Work out the finished part from the listing and answer in its coordinate system (mm). A direction names the side the tool comes from. Round coordinates to 2 decimals unless told otherwise and drop trailing zeros. Loops run counter-clockwise (first coordinate to the right, second up) from the corner with the lowest first, then second, coordinate; pieces in that order, holes last. Notation, with made-up numbers: (6.25, -30.5) - (53.25, -30.5) arc R20 cw to (53.25, -22.5) - close; hole circle Ø3 at (-35.5, 17). An arc over 180 degrees is marked (long way). Answer as CSV lines item,"result". Start each with the question number.
Q1. Straight lines are drawn through the part: L1, parallel to Y at x = 5, z = -14.05; L2, parallel to X at y = 10.5, z = -11; L3, parallel to Z at x = 2.75, y = 6.75. For each, find the intervals that lie inside material, in ascending order. Write a range as [from, to].
Q2. Section A-A on x = 5 is taken. Write down the section's boundary in (y, z).
Q3. Each of these flat-tipped pins is pushed along its axis until it touches: pin 1 Ø4.5 at (x, z) = (5.5, -9) entering from -Y; pin 2 Ø2.5 at (x, z) = (5, -11) entering from +Y; pin 3 Ø2 at (y, z) = (12, -6) entering from -X; pin 4 Ø1.2 at (x, y) = (5, 12) entering from -Z. Where does it stop, or does it pass through?
Q4. Section B-B on z = -11 is taken. Write down the section's boundary in (x, y).
Q5. For faces 5 (the face through (9.699, 10.126, 0.285)), 6 (the face through (5, 9, -8)), 7 (the face through (9.715, 10.126, 29.699)), 8 (the face through (2, 12, -8)), 9 (the face through (7.715, 9.301, -8.098)), determine the directions among +Z, -Z, +X, -X, +Y, -Y from which every point of the face is accessible in a straight line to the end or side of a thin tool.
Q6. The mould has two halves that part along X. Classify faces 1 (the face through (6, 12, -14)), 2 (the face through (2, 8, 0)), 3 (the face through (0.285, 10.126, 29.699)), 4 (the face through (5.07, 11.96, -9.5)): +X half, -X half, draft (parallel to the pull), parting line (faces both ways), or undercut.
Q7. Section D-D on y = 5.75 is taken. Write down the section's boundary in (x, z).
```python
from build123d import *

# Parameters (mm, degrees)
SKETCH_1_W          = 10
SKETCH_1_H          = 22
EXTRUDE_1_DEPTH     = 30
SKETCH_2_W          = 6
SKETCH_2_H          = 6
EXTRUDE_3_DEPTH     = 14
SKETCH_3_R          = 1.5
CUT_EXTRUDE_1_DEPTH = 6
SKETCH_6_W          = 10
SKETCH_6_H          = 30
CUT_EXTRUDE_2_DEPTH = 2
SKETCH_7_W          = 6
SKETCH_7_H          = 6
EXTRUDE_4_DEPTH     = 2
SKETCH_8_R          = 1
CUT_EXTRUDE_3_DEPTH = 4
FILLET_1_R          = 1


with BuildPart() as part:
    # 草图1 → 凸台-拉伸1 (new body)
    with BuildSketch(Plane.XY):
        with Locations((5, 11)):
            Rectangle(SKETCH_1_W, SKETCH_1_H)
    extrude(amount=EXTRUDE_1_DEPTH)

    # 草图2 → 凸台-拉伸3 (add)
    with BuildSketch(Plane.XY):
        with Locations((5, 12)):
            Rectangle(SKETCH_2_W, SKETCH_2_H)
    extrude(amount=-EXTRUDE_3_DEPTH)

    # 草图3 → 切除-拉伸1 (cut)
    with BuildSketch(Plane(origin=(0, 9, 0), x_dir=(-1, 0, 0), z_dir=(0, -1, 0))):
        with Locations(Location((-5, 11, 0), (0, 0, 90))):
            Circle(SKETCH_3_R)
    extrude(amount=-CUT_EXTRUDE_1_DEPTH, mode=Mode.SUBTRACT)

    # 草图6 → 切除-拉伸2 (cut)
    with BuildSketch(Plane(origin=(0, 22, 0), x_dir=(1, 0, 0), z_dir=(0, 1, 0))):
        with Locations((5, -15)):
            Rectangle(SKETCH_6_W, SKETCH_6_H)
    extrude(amount=-CUT_EXTRUDE_2_DEPTH, mode=Mode.SUBTRACT)

    # 草图7 → 凸台-拉伸4 (add)
    with BuildSketch(Plane(origin=(0, 0, -14), x_dir=(-1, 0, 0), z_dir=(0, 0, -1))):
        with Locations((-5, 12)):
            Rectangle(SKETCH_7_W, SKETCH_7_H)
    extrude(amount=EXTRUDE_4_DEPTH)

    # 草图8 → 切除-拉伸3 (cut)
    with BuildSketch(Plane(origin=(0, 0, -16), x_dir=(-1, 0, 0), z_dir=(0, 0, -1))):
        with Locations((-5, 12)):
            Circle(SKETCH_8_R)
    extrude(amount=-CUT_EXTRUDE_3_DEPTH, mode=Mode.SUBTRACT)

    # 圆角1
    fillet_1_edges = [part.edges().sort_by_distance(p)[0] for p in [
        (10, 10, 30),
        (2, 9, -8),
        (2, 15, -8),
        (8, 15, -8),
        (8, 9, -8),
        (2, 12, 0),
        (5, 9, 0),
        (8, 12, 0),
        (5, 15, 0),
        (0, 10, 30),
        (0, 10, 0),
        (0, 20, 15),
        (5, 20, 0),
        (10, 20, 15),
        (5, 20, 30),
        (2, 12, -16),
        (5, 15, -16),
        (8, 12, -16),
        (5, 9, -16),
        (10, 10, 0),
        (5, 0, 0),
        (10, 0, 15),
        (0, 0, 15),
        (5, 0, 30),
    ]]
    fillet(fillet_1_edges, radius=FILLET_1_R - 0.0001)  # a hair under: the kernel refuses the full size


solid = part.part
```
Findings:
1,L1,"y = [9, 11], [13, 15]"
1,L2,"x = [2, 3.5], [6.5, 8]"
1,L3,"z = [0, 30]"
2,outline,"(0, 1) arc R1 ccw to (1, 0) - (8, 0) arc R1 cw to (9, -1) - (9, -9.5) - (15, -9.5) - (15, -1) arc R1 cw to (16, 0) - (19, 0) arc R1 ccw to (20, 1) - (20, 29) arc R1 ccw to (19, 30) - (1, 30) arc R1 ccw to (0, 29) - close; (9, -15) arc R1 ccw to (10, -16) - (11, -16) - (11, -12.5) - (9, -12.5) - close; (13, -16) - (14, -16) arc R1 ccw to (15, -15) - (15, -12.5) - (13, -12.5) - close"
3,pin 1,"stops at y = 9"
3,pin 2,"passes through"
3,pin 3,"stops at x = 2"
3,pin 4,"stops at z = -9.63"
4,outline,"(2, 10) arc R1 ccw to (3, 9) - (3.5, 9) - (3.5, 15) - (3, 15) arc R1 ccw to (2, 14) - close; (6.5, 9) - (7, 9) arc R1 ccw to (8, 10) - (8, 14) arc R1 ccw to (7, 15) - (6.5, 15) - close"
5,face 5,"-Z, +X, +Y, -Y"
5,face 6,"-Z, +X, -X, -Y"
5,face 7,"+Z, +X, +Y, -Y"
5,face 8,"-Z, -X, +Y, -Y"
5,face 9,"-Z, +X, -Y"
6,face 1,"undercut"
6,face 2,"draft"
6,face 3,"-X half"
6,face 4,"undercut"
7,outline,"(0, 1) arc R1 ccw to (1, 0) - (9, 0) arc R1 ccw to (10, 1) - (10, 29) arc R1 ccw to (9, 30) - (1, 30) arc R1 ccw to (0, 29) - close"
